Geometry check sheet. Reference: the model listing, model coordinates, mm. A direction names the side the tool comes from. Give positions to 0.01 mm unless a question says otherwise; leave off trailing zeros. Write each loop counter-clockwise with the first axis right and the second up, starting at its lowest first coordinate (ties: lowest second). Pieces come first, ordered by that corner, then holes. Notation, with made-up numbers: (80, 10) - (116, 10) arc R30 cw to (116, 36) - close; hole circle Ø2 at (68.5, 62). An arc over 180 degrees is marked (long way). One line per question, with ' | ' between items. Start each with the question number.
Q1. Thickness scan on L1, parallel to Z at x = 104, y = -336; L2, parallel to Z at x = -42, y = -2207.5; L3, parallel to X at y = -543, z = -15. Record the ranges inside material, lowest first. Write a range as [from, to].
Q2. Section check B-B on y = -1435.5. Record the boundary of the cut face in (x, z), and give its area (3 significant figures).
Q3. Gauge pin test, flat ends, axial feed: P1, Ø1.6, axis at y = -2419.5, z = 24, coming from the +X side; P2, Ø3, axis at y = -372.5, z = 12.5, coming from the -X side; P3, Ø12, axis at x = 70.5, z = 17.5, coming from the -Y side; P4, Ø3, axis at y = -645.5, z = 19, coming from the +X side. Record the tip position at first contact, or that the pin passes through.
Q4. Release check for a two-part mould opening along X. For faces 3 (the face through (110, -1233, 22.348)), 4 (the face through (-53.14, -1232.5, 3.94)), 5 (the face through (52.34, -1232.5, 2.38)), 6 (the face through (50.76, -1232.5, 4.93)) record: +X half, -X half, draft (parallel to the pull), parting line (faces both ways), or undercut.
Q5. Section check C-C on x = 6. Record the boundary of the cut face in (y, z).
Q6. Section check A-A on z = 14.5. Record the boundary of the cut face in (x, y), and give its area (3 significant figures).
Q7. Set-up check for faces 1 (the face through (-1, -1232, -17.044)), 2 (the face through (0, -1232, -15.044)): record each of +Z, -Z, +X, -X, +Y, -Y from which the full face is reachable in a straight line by a thin tool's end or side.
```python
from build123d import *

# Parameters (mm, degrees)
F1_DEPTH = 2500
F2_DEPTH = 50
F3_W     = 60.1930970593
F3_H     = 2
F4_DEPTH = 275


with BuildPart() as f1:
    # F0 (on Front) → F1 (new body)
    with BuildSketch(Plane.XZ):
        Polygon((-47.7612030406, -15.0440340683), (-54.7071301473, 24.3482760522), (-56.7379833711, 24.3482760522), (-49.439402303, -17.0440340683), (48.9169962217, -17.0440340683), (55.8629233284, 22.3482760522), (115.8629233284, 22.3482760522), (115.8629233284, 24.3482760522), (54.1847240661, 24.3482760522), (47.2387969594, -15.0440340683), align=None)
    extrude(amount=F1_DEPTH)

    # F2 (add): a face of the model
    f2_faces = [f1.faces().sort_by_distance(p)[0] for p in [
        (115.8629233284, -1250, 23.3482760522),
    ]]
    extrude(f2_faces, amount=F2_DEPTH)

    # F3 (on face) → F4 (cut)
    with BuildSketch(Plane.XZ.offset(2500)):
        with Locations((135.7663747988, 23.3482760522)):
            Rectangle(F3_W, F3_H)
    extrude(amount=-F4_DEPTH, mode=Mode.SUBTRACT)


solid = f1.part
```
Working result:
1) L1: z = [22.35, 24.35] | L2: z = [-17.04, -15.04] | L3: x = [-49.8, -47.77], [47.25, 49.28]
2) outline: (-56.74, 24.35) - (-49.44, -17.04) - (48.92, -17.04) - (55.86, 22.35) - (165.86, 22.35) - (165.86, 24.35) - (54.18, 24.35) - (47.24, -15.04) - (-47.76, -15.04) - (-54.71, 24.35) - close | area: 577 mm2
3) P1: stops at x = 105.67 | P2: stops at x = -54.91 | P3: stops at y = -2500 | P4: stops at x = 55.54
4) face 3: draft | face 4: -X half | face 5: +X half | face 6: undercut
5) outline: (-2500, -17.04) - (0, -17.04) - (0, -15.04) - (-2500, -15.04) - close
6) outline: (-55, -2500) - (-52.97, -2500) - (-52.97, 0) - (-55, 0) - close; (52.45, -2500) - (54.48, -2500) - (54.48, 0) - (52.45, 0) - close | area: 10,200 mm2
7) face 1: -Z, +X, -X, +Y, -Y | face 2: +Z, +Y, -Y
